```python
from build123d import *

# Parameters (mm, degrees)
F3_W         = 27
F3_H         = 27
F4_DEPTH     = 30
F5_T1_DEPTH  = 607
F5_T3_DEPTH  = 772
F5_T5_DEPTH  = 808
F5_T7_DEPTH  = 643
F5_T13_DEPTH = 777
F5_T17_DEPTH = 612
F5_T20_DEPTH = 617
F5_T22_DEPTH = 782
F5_T24_DEPTH = 820
F5_T26_DEPTH = 775
F5_T28_DEPTH = 610
F5_T30_DEPTH = 655
F5_T36_DEPTH = 780
F5_T40_DEPTH = 615
F5_T47_DEPTH = 780
F5_T51_DEPTH = 615


# Not quite as in the source:
# - a fillet or chamfer that OpenCascade refuses, or shapes differently, is made with other operations: its cross-section is extruded or revolved along the edge and cut away or added


with BuildPart() as f2:
    # F2: sweep along a path in F1
    with BuildLine(Plane.XY) as f2_path:
        Line((0, 0), (0, 770))
        Line((0, 770), (605, 770))
    # F0 (on Front) → F2 (sweep)
    with BuildSketch(Plane.XZ):
        Polygon((0, -350), (0, 0), (-40, 0), (-40, -25), (-38, -25), (-38, -2), (-2, -2), (-2, -348), (-29, -348), (-29, -376), (-27, -376), (-27, -350), align=None)
    sweep(path=f2_path.line, transition=Transition.RIGHT)

    # F3 (on face) → F4 (cut)
    with BuildSketch(Plane.XY.offset(-348)):
        with Locations((-15.5, 785.5)):
            Rectangle(F3_W, F3_H)
    extrude(amount=-F4_DEPTH, mode=Mode.SUBTRACT)

    # F5: fillet of radius 2 on 15 edges, made by hand

    # F5_s2 → F5_t1 (join)
    with BuildSketch(Plane.YZ.offset(-2)):
        with BuildLine():
            ThreePointArc((774, -348), (772.5857864376, -347.4142135624), (772, -346))
            Line((772, -346), (772, -348))
            Line((772, -348), (774, -348))
        make_face()
        with BuildLine():
            ThreePointArc((774, -2), (772.5857864376, -2.5857864376), (772, -4))
            Line((772, -4), (772, -2))
            Line((772, -2), (774, -2))
        make_face()
        with BuildLine():
            ThreePointArc((795, -350), (796.4142135624, -350.5857864376), (797, -352))
            Line((797, -352), (797, -350))
            Line((797, -350), (795, -350))
        make_face()
    extrude(amount=F5_T1_DEPTH)

    # F5_s4 → F5_t3 (join)
    with BuildSketch(Plane.XZ.offset(-772)):
        with BuildLine():
            ThreePointArc((-4, -2), (-2.5857864376, -2.5857864376), (-2, -4))
            Line((-2, -4), (-2, -2))
            Line((-2, -2), (-4, -2))
        make_face()
        with BuildLine():
            ThreePointArc((-25, -350), (-26.4142135624, -350.5857864376), (-27, -352))
            Line((-27, -352), (-27, -350))
            Line((-27, -350), (-25, -350))
        make_face()
    extrude(amount=F5_T3_DEPTH)

    # F5_s6 → F5_t5 (join)
    with BuildSketch(Plane.XZ.offset(-808)):
        with BuildLine():
            ThreePointArc((-38, -4), (-37.4142135624, -2.5857864376), (-36, -2))
            Line((-36, -2), (-38, -2))
            Line((-38, -2), (-38, -4))
        make_face()
    extrude(amount=F5_T5_DEPTH)

    # F5_s8 → F5_t7 (join)
    with BuildSketch(Plane.YZ.offset(-38)):
        with BuildLine():
            ThreePointArc((806, -2), (807.4142135624, -2.5857864376), (808, -4))
            Line((808, -4), (808, -2))
            Line((808, -2), (806, -2))
        make_face()
    extrude(amount=F5_T7_DEPTH)


with BuildPart() as f5_tool11:
    # F5_s12 → F5_t13 (new body)
    with BuildSketch(Plane.XZ):
        with BuildLine():
            ThreePointArc((-4, -2), (-2.5857864376, -2.5857864376), (-2, -4))
            Line((-2, -4), (-2, -2))
            Line((-2, -2), (-4, -2))
        make_face()
    extrude(amount=-F5_T13_DEPTH)

    split(bisect_by=Plane.XZ.offset(-772), keep=Keep.BOTTOM)


with BuildPart() as f5_tool15:
    # F5_s16 → F5_t17 (new body)
    with BuildSketch(Plane.YZ.offset(-7)):
        with BuildLine():
            ThreePointArc((774, -2), (772.5857864376, -2.5857864376), (772, -4))
            Line((772, -4), (772, -2))
            Line((772, -2), (774, -2))
        make_face()
    extrude(amount=F5_T17_DEPTH)

    split(bisect_by=Plane.YZ.offset(-2), keep=Keep.BOTTOM)


with BuildPart() as f5_tool11_1:
    add(f5_tool11.part)

    # F5_t19: intersect F5_tool15
    add(f5_tool15.part, mode=Mode.INTERSECT)


with BuildPart() as f2_1:
    add(f2.part)

    # F5_t9: union F5_tool11
    add(f5_tool11_1.part)

    # F5_s21 → F5_t20 (cut)
    with BuildSketch(Plane.YZ.offset(-7)):
        with BuildLine():
            ThreePointArc((799, -350), (798.4142135624, -348.5857864376), (797, -348))
            Line((797, -348), (799, -348))
            Line((799, -348), (799, -350))
        make_face()
    extrude(amount=F5_T20_DEPTH, mode=Mode.SUBTRACT)

    # F5_s23 → F5_t22 (cut)
    with BuildSketch(Plane.XZ.offset(-777)):
        with BuildLine():
            ThreePointArc((-29, -350), (-28.4142135624, -348.5857864376), (-27, -348))
            Line((-27, -348), (-29, -348))
            Line((-29, -348), (-29, -350))
        make_face()
    extrude(amount=F5_T22_DEPTH, mode=Mode.SUBTRACT)

    # F5_s25 → F5_t24 (cut)
    with BuildSketch(Plane.XZ.offset(-815)):
        with BuildLine():
            ThreePointArc((-40, -2), (-39.4142135624, -0.5857864376), (-38, 0))
            Line((-38, 0), (-40, 0))
            Line((-40, 0), (-40, -2))
        make_face()
    extrude(amount=F5_T24_DEPTH, mode=Mode.SUBTRACT)

    # F5_s27 → F5_t26 (cut)
    with BuildSketch(Plane.XZ.offset(-770)):
        with BuildLine():
            ThreePointArc((0, -2), (-0.5857864376, -0.5857864376), (-2, 0))
            Line((-2, 0), (0, 0))
            Line((0, 0), (0, -2))
        make_face()
        with BuildLine():
            ThreePointArc((0, -348), (-0.5857864376, -349.4142135624), (-2, -350))
            Line((-2, -350), (0, -350))
            Line((0, -350), (0, -348))
        make_face()
    extrude(amount=F5_T26_DEPTH, mode=Mode.SUBTRACT)

    # F5_s29 → F5_t28 (cut)
    with BuildSketch(Plane.YZ):
        with BuildLine():
            ThreePointArc((770, -2), (770.5857864376, -0.5857864376), (772, 0))
            Line((772, 0), (770, 0))
            Line((770, 0), (770, -2))
        make_face()
        with BuildLine():
            ThreePointArc((770, -348), (770.5857864376, -349.4142135624), (772, -350))
            Line((772, -350), (770, -350))
            Line((770, -350), (770, -348))
        make_face()
    extrude(amount=F5_T28_DEPTH, mode=Mode.SUBTRACT)

    # F5_s31 → F5_t30 (cut)
    with BuildSketch(Plane.YZ.offset(-45)):
        with BuildLine():
            ThreePointArc((810, -2), (809.4142135624, -0.5857864376), (808, 0))
            Line((808, 0), (810, 0))
            Line((810, 0), (810, -2))
        make_face()
    extrude(amount=F5_T30_DEPTH, mode=Mode.SUBTRACT)


with BuildPart() as f5_tool34:
    # F5_s35 → F5_t36 (new body)
    with BuildSketch(Plane.XZ.offset(5)):
        with BuildLine():
            ThreePointArc((0, -2), (-0.5857864376, -0.5857864376), (-2, 0))
            Line((-2, 0), (0, 0))
            Line((0, 0), (0, -2))
        make_face()
    extrude(amount=-F5_T36_DEPTH)

    split(bisect_by=Plane.XZ.offset(-770), keep=Keep.BOTTOM)


with BuildPart() as f5_tool38:
    # F5_s39 → F5_t40 (new body)
    with BuildSketch(Plane.YZ.offset(-5)):
        with BuildLine():
            ThreePointArc((770, -2), (770.5857864376, -0.5857864376), (772, 0))
            Line((772, 0), (770, 0))
            Line((770, 0), (770, -2))
        make_face()
    extrude(amount=F5_T40_DEPTH)

    split(bisect_by=Plane.YZ, keep=Keep.BOTTOM)


with BuildPart() as f5_tool34_1:
    add(f5_tool34.part)

    # F5_t42: intersect F5_tool38
    add(f5_tool38.part, mode=Mode.INTERSECT)


with BuildPart() as f2_2:
    add(f2_1.part)

    # F5_t32: cut F5_tool34
    add(f5_tool34_1.part, mode=Mode.SUBTRACT)


with BuildPart() as f5_tool45:
    # F5_s46 → F5_t47 (new body)
    with BuildSketch(Plane.XZ.offset(5)):
        with BuildLine():
            ThreePointArc((0, -348), (-0.5857864376, -349.4142135624), (-2, -350))
            Line((-2, -350), (0, -350))
            Line((0, -350), (0, -348))
        make_face()
    extrude(amount=-F5_T47_DEPTH)

    split(bisect_by=Plane.XZ.offset(-770), keep=Keep.BOTTOM)


with BuildPart() as f5_tool49:
    # F5_s50 → F5_t51 (new body)
    with BuildSketch(Plane.YZ.offset(-5)):
        with BuildLine():
            ThreePointArc((770, -348), (770.5857864376, -349.4142135624), (772, -350))
            Line((772, -350), (770, -350))
            Line((770, -350), (770, -348))
        make_face()
    extrude(amount=F5_T51_DEPTH)

    split(bisect_by=Plane.YZ, keep=Keep.BOTTOM)


with BuildPart() as f5_tool45_1:
    add(f5_tool45.part)

    # F5_t53: intersect F5_tool49
    add(f5_tool49.part, mode=Mode.INTERSECT)


with BuildPart() as f2_3:
    add(f2_2.part)

    # F5_t43: cut F5_tool45
    add(f5_tool45_1.part, mode=Mode.SUBTRACT)


solid = f2_3.part
```
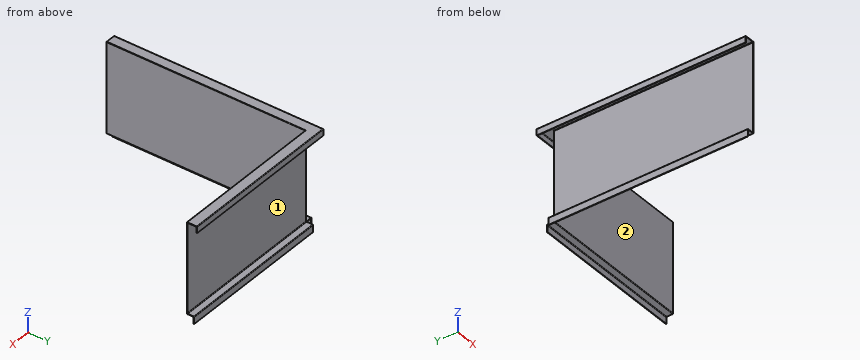
The listing builds one solid part. Answer for the finished solid, in the listing's coordinates (mm). Face numbers are marked on the shaded views. Give positions to 0.01 mm unless a question says otherwise; leave off trailing zeros. Write each loop counter-clockwise with the first axis right and the second up, starting at its lowest first coordinate (ties: lowest second). Pieces come first, ordered by that corner, then holes. Notation, with made-up numbers: (-13.75, -14.5) -> (-0.75, -14.5) arc R28 cw to (-0.75, 21.5) -> close; hole circle Ø9 at (52, 36). An arc over 180 degrees is marked (long way). Use one line per item in the form item = value.
1) Section B-B on x = 500.5 is taken. Write down the section's boundary in (y, z), plus the area to 3 significant figures.
Result:
outline = (770, -348) arc R2 ccw to (772, -350) -> (795, -350) arc R2 cw to (797, -352) -> (797, -376) -> (799, -376) -> (799, -350) arc R2 ccw to (797, -348) -> (774, -348) arc R2 cw to (772, -346) -> (772, -4) arc R2 cw to (774, -2) -> (806, -2) arc R2 cw to (808, -4) -> (808, -25) -> (810, -25) -> (810, -2) arc R2 ccw to (808, 0) -> (772, 0) arc R2 ccw to (770, -2) -> close
area = 928 mm²
2) Each of these flat-tipped pins is pushed along its axis until it touches: P1, Ø21, axis at x = 171.5, z = -366, coming from the +Y side; P2, Ø23, axis at x = 220.5, z = -14, coming from the -Y side; P3, Ø6.5, axis at y = 241, z = -16.5, coming from the +X side. Where does it stop, or does it pass through?
Result:
P1 = 799
P2 = 770
P3 = 0
3) For a pull along Z with two mould halves and no side action, classify the marked faces 1 and 2 as +Z half, -Z half, draft (parallel to the pull), parting line (faces both ways), or undercut.
Result:
face_1 = undercut
face_2 = draft
4) Section C-C on z = -145 is taken. Write down the section's boundary in (x, y).
Result:
outline = (-2, 0) -> (0, 0) -> (0, 770) -> (605, 770) -> (605, 772) -> (-2, 772) -> close
5) Straight lines are drawn through the part: probe 1 along X at (y, z) = (176, -16.5); probe 2 along Y at (x, z) = (493.5, -20); probe 3 along X at (y, z) = (313, -254). For each, find the intervals that lie inside material, in ascending order.
Result:
probe_1 = -40 to -38, -2 to 0
probe_2 = 770 to 772, 808 to 810
probe_3 = -2 to 0
6) Section A-A on y = 418 is taken. Write down the section's boundary in (x, z), plus the area to 3 significant figures.
Result:
outline = (-40, -25) -> (-38, -25) -> (-38, -4) arc R2 cw to (-36, -2) -> (-4, -2) arc R2 cw to (-2, -4) -> (-2, -348) -> (-27, -348) arc R2 ccw to (-29, -350) -> (-29, -376) -> (-27, -376) -> (-27, -352) arc R2 cw to (-25, -350) -> (-2, -350) arc R2 ccw to (0, -348) -> (0, -2) arc R2 ccw to (-2, 0) -> (-38, 0) arc R2 ccw to (-40, -2) -> close
area = 927 mm²
